```python
from build123d import *

# Parameters (mm, degrees)
SKETCH1_R           = 6.395
BOSS_EXTRUDE1_DEPTH = 80.99
SKETCH3_W           = 6.14
SKETCH3_H           = 3.7
CUT_EXTRUDE2_DEPTH  = 8.5
CUT_EXTRUDE3_DEPTH  = 1.28
CIRPATTERN1_COUNT   = 4


with BuildPart() as part:
    # Sketch1 → Boss-Extrude1 (new body)
    with BuildSketch(Plane(origin=(0, 0, 0), x_dir=(1, 0, 0), z_dir=(0, 1, 0))):
        Circle(SKETCH1_R)
    extrude(amount=BOSS_EXTRUDE1_DEPTH)

    # Sketch3 → Cut-Extrude2 (cut)
    with BuildSketch(Plane.XZ):
        Rectangle(SKETCH3_W, SKETCH3_H)
    extrude(amount=-CUT_EXTRUDE2_DEPTH, mode=Mode.SUBTRACT)

    # Sketch4 → Cut-Extrude3 (cut)
    with BuildSketch(Plane(origin=(-0.091269963, 0, 0.633458597), x_dir=(0.989779057, 0, 0.142609318), z_dir=(-0.142609318, 0, 0.989779057))):
        Polygon((-3.84099181, 80.99), (-6.12099181, 80.99), (-6.12099181, 79.513663006), (-3.84099181, 80.733663006), align=None)
    cut_extrude3 = extrude(amount=-CUT_EXTRUDE3_DEPTH, mode=Mode.SUBTRACT)

    # CirPattern1: Cut-Extrude3 ×4 about axis
    cirpattern1_axis = Axis((0, 0, 0), (0, 1, 0))
    for i in range(1, CIRPATTERN1_COUNT):
        add(cut_extrude3.rotate(cirpattern1_axis, i * 360 / CIRPATTERN1_COUNT), mode=Mode.SUBTRACT)


solid = part.part
```
For this review, take the finished solid that the model builds, in its own axes (mm). A direction names the side the tool comes from. Coordinates: 2 decimals unless noted, no trailing zeros. Loops run counter-clockwise (first coordinate to the right, second up) from the corner with the lowest first, then second, coordinate; pieces in that order, holes last. Notation, with made-up numbers: (70, 43.25) -> (77, 43.25) arc R35 ccw to (77, 76.25) -> close; hole circle Ø4 at (18.5, 56.5). An arc over 180 degrees is marked (long way). Return JSON: item names as keys, results as strings. Group by question number.
(1) Mouldability with a two-part tool opening along Z and no side actions: class faces 4 (the cylindrical face through (-0.83, 39.93, -6.34)), 5 (the flat face through (0, 80.99, 0)), 6 (the flat face through (-6.06, 80.26, -0.86)) as pulls with the +Z half, pulls with the -Z half, needs draft (parallel to the pull), parting line crosses it, or undercut.
(2) Consider section A-A, the plane y = 60. Give the boundary of the cut face in (x, z) (3 decimals), plus the area to 3 significant figures.
(3) Consider section B-B, the plane z = -3. Give the boundary of the cut face in (x, y).
(4) For pin 1 Ø1.8 at (x, z) = (0, 0) entering from -Y; pin 2 Ø2 at (y, z) = (9, 2) entering from +X; pin 3 Ø6 at (y, z) = (13, 4) entering from -X, all flat-tipped, find the tip position at first contact; note any pin that passes through.
(5) Tool access review of faces 1 (the flat face through (0, 8.5, 0)), 2 (the flat face through (0.115, 80.426, -5.288)), 3 (the flat face through (0, 0, 3)): name each direction out of +Z, -Z, +X, -X, +Y, -Y from which nothing blocks a thin tool from reaching the whole face with its end or side.
(6) To check wall thickness, follow L1, parallel to Z at x = 1.75, y = 10.5; L2, parallel to Y at x = 0, z = 1. State the ranges of each line that lie inside material, in increasing order.
Results below:
{
 "1": {"face 4": "parting line crosses it", "face 5": "needs draft", "face 6": "undercut"},
 "2": {"outline": "circle Ø12.79 at (0, 0)", "area": "128 mm2"},
 "3": {"outline": "(-5.65, 0) -> (5.65, 0) -> (5.65, 80.99) -> (-5.65, 80.99) -> close"},
 "4": {"pin 1": "stops at y = 8.5", "pin 2": "stops at x = 6.32", "pin 3": "stops at x = -6.32"},
 "5": {"face 1": "-Y", "face 2": "+Y", "face 3": "+Z, -Z, +X, -X, -Y"},
 "6": {"L1": "z = -6.15 to 6.15", "L2": "y = 8.5 to 80.99"}
}
